Read the model definition and answer for the solid it produces. Units are mm, in the model's axes. Face numbers are marked on the shaded views. A direction names the side the tool comes from. Coordinates: 2 decimals unless noted, no trailing zeros. Order: outer loops, then holes, each group sorted by start corner. A loop starts at its lowest first (then second) coordinate and runs counter-clockwise, first axis right, second up. Notation, with made-up numbers: M -17.5,6.5 L -10.5,6.5 A24 cw -10.5,22.5 Z; hole C 45,-29 d8. An arc over 180 degrees is marked long. Use a Markdown table: item, result. Add a question column.
1) Find section A-A on y = -11. Write down the section's boundary in (x, z).
2) The mould has two halves that part along Z. Classify the marked faces 4, 5 and 6: released by +Z, released by -Z, zero draft, split by the parting line, or undercut.
3) Find section B-B on y = -0.5. Write down the section's boundary in (x, z) (3 decimals).
4) Find the intervals of material crossed by probe 1 along X at (y, z) = (-14.5, 0); probe 2 along Z at (x, y) = (0.25, -16.5); probe 3 along Z at (x, y) = (1, -7), in increasing order. Write a range as [from, to].
5) For the marked faces 1, 2 and 3, determine the directions among +Z, -Z, +X, -X, +Y, -Y from which every point of the face is accessible in a straight line to the end or side of a thin tool.
6) Each of these flat-tipped pins is pushed along its axis until it touches: pin 1 Ø6 at (x, z) = (2.5, -6) entering from -Y; pin 2 Ø2.5 at (x, z) = (-5, -5) entering from +Y; pin 3 Ø3 at (x, z) = (-1.5, 8) entering from -Y; pin 4 Ø1.8 at (x, z) = (3.5, -5.5) entering from -Y. Where does it stop, or does it pass through?
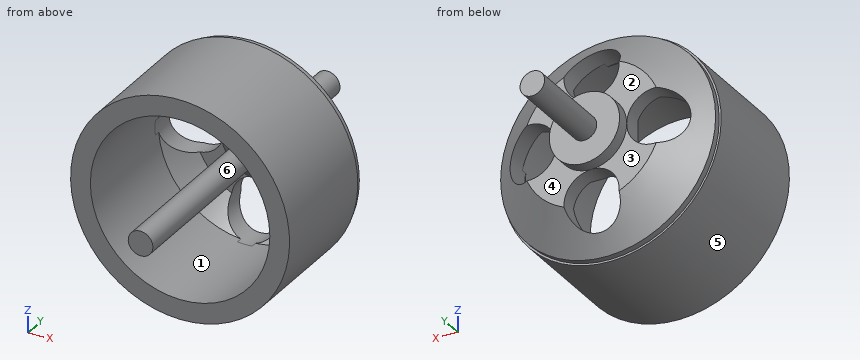
from build123d import *

# Parameters (mm, degrees)
SKETCH3_R          = 13.843
SKETCH3_R_2        = 1.55575
CUT_EXTRUDE2_DEPTH = 38.213955992
SKETCH2_R          = 3.4925
CUT_EXTRUDE1_DEPTH = 5.08


with BuildPart() as part:
    # Sketch1 → Revolve1 (revolve)
    with BuildSketch(Plane.XY, mode=Mode.PRIVATE) as revolve1_sk:
        Polygon((0, 11.176), (1.55575, 11.176), (1.55575, 0), (4.445, 0), (4.445, -1.524), (8.89, -1.524), (13.589, -5.08), (13.589, -5.842), (13.843, -5.842), (13.843, -20.4724), (13.589, -20.4724), (13.589, -23.0124), (12.7, -26.67), (3.81, -26.67), (3.81, -26.924), (1.55575, -26.924), (1.55575, -28.956), (0, -28.956), align=None)
    revolve(revolve1_sk.sketch.rotate(Axis((0, -28.956, 0), (0, 1, 0)), 90), axis=Axis((0, -28.956, 0), (0, 1, 0)))

    # Sketch3 → Cut-Extrude2 (cut, through all)
    with BuildSketch(Plane.XZ.offset(20.4724)):
        with Locations(Location((0, 0, 0), (0, 0, 270))):
            Circle(SKETCH3_R)
        with Locations(Location((0, 0, 0), (0, 0, 270))):
            Circle(SKETCH3_R_2, mode=Mode.SUBTRACT)
    extrude(amount=CUT_EXTRUDE2_DEPTH, mode=Mode.SUBTRACT)

    # Sketch5 → Cut-Revolve1 (revolve, cut)
    with BuildSketch(Plane.XY, mode=Mode.PRIVATE) as cut_revolve1_sk:
        Polygon((11.343, -5.888455731), (11.343, -24.765583443), (1.55575, -24.765583443), (1.55575, -5.842), (2.55575, -5.842), (4.87375, -3.524), (8.218540641, -3.524), align=None)
    revolve(cut_revolve1_sk.sketch.rotate(Axis((0, 11.176, 0), (0, -1, 0)), 90), axis=Axis((0, 11.176, 0), (0, -1, 0)), mode=Mode.SUBTRACT)

    # Sketch2 → Cut-Extrude1 (cut)
    with BuildSketch(Plane(origin=(0, -1.524, 0), x_dir=(1, 0, 0), z_dir=(0, 1, 0))):
        with Locations(Location((0, 7.9375, 0), (0, 0, 270))):
            Circle(SKETCH2_R)
        with Locations(Location((7.9375, 0, 0), (0, 0, 273.961773505))):
            Circle(SKETCH2_R)
        with Locations(Location((0, -7.9375, 0), (0, 0, 90))):
            Circle(SKETCH2_R)
        with Locations(Location((-7.9375, 0, 0), (0, 0, 266.038226276))):
            Circle(SKETCH2_R)
    extrude(amount=-CUT_EXTRUDE1_DEPTH, mode=Mode.SUBTRACT)


solid = part.part
Check result:
| question | item | result |
|---|---|---|
| 1 | outline | C 0,0 d27.69; C 0,0 d3.11; hole C 0,0 d22.69 |
| 2 | face 4 | zero draft |
| 2 | face 5 | split by the parting line |
| 2 | face 6 | undercut |
| 3 | outline | C 0,0 d8.89 |
| 4 | probe 1 | x = [-13.84, -11.34], [-1.56, 1.56], [11.34, 13.84] |
| 4 | probe 2 | z = [-13.84, -11.34], [-1.54, 1.54], [11.34, 13.84] |
| 4 | probe 3 | z = [-13.81, -11.3], [-1.19, 1.19], [11.3, 13.81] |
| 5 | face 1 | -Y |
| 5 | face 2 | +Z, -X, +Y |
| 5 | face 3 | -Z, -X, +Y |
| 6 | pin 1 | stops at y = -4.9 |
| 6 | pin 2 | stops at y = -1.52 |
| 6 | pin 3 | passes through |
| 6 | pin 4 | stops at y = -3.52 |
